Read the model definition and answer for the solid it produces. Units are mm, in the model's axes. Coordinates: 2 decimals unless noted, no trailing zeros. Order: outer loops, then holes, each group sorted by start corner. A loop starts at its lowest first (then second) coordinate and runs counter-clockwise, first axis right, second up.
from build123d import *

# Parameters (mm, degrees)
SKETCH1_W           = 30
SKETCH1_H           = 75.2
SKETCH1_R           = 5.25
BOSS_EXTRUDE1_DEPTH = 2.5
FILLET1_R           = 2


with BuildPart() as part:
    # Sketch1 → Boss-Extrude1 (new, symmetric)
    with BuildSketch(Plane.XY):
        Rectangle(SKETCH1_W, SKETCH1_H)
        with Locations((0, 23.1)):
            Circle(SKETCH1_R, mode=Mode.SUBTRACT)
    extrude(amount=BOSS_EXTRUDE1_DEPTH, both=True)

    # Fillet1
    fillet1_edges = [part.edges().sort_by_distance(p)[0] for p in [
        (-15, 37.6, 0),
        (15, 37.6, 0),
    ]]
    fillet(fillet1_edges, radius=FILLET1_R)


solid = part.part
Q1. This flat-tipped pin is pushed along its axis until it touches: P1, Ø6, axis at x = -1.5, y = 24, coming from the -Z side. Where does it stop, or does it pass through?
Q2. The part is cut by section C-C, the plane x = 0. Determine the outline of the cut face in (y, z).
Q3. Determine the mould class of faces 1 (the cylindrical face through (2.82, 27.53, -0.04)), 2 (the flat face through (0, 1, 2.5)), 3 (the cylindrical face through (14.43, 37, -0.04)) for opening direction X: +X half, -X half, draft (parallel to the pull), parting line (faces both ways), or undercut.
Q4. Straight lines are drawn through the part: L1, parallel to Y at x = 0, z = -0.25; L2, parallel to Y at x = -2.75, z = -1.6. For each, find the intervals that lie inside material, in ascending order.
Q5. The part is cut by section A-A, the plane z = -0.15. Determine the outline of the cut face in (x, y), then the cut area to 3 significant figures.
Q6. The part is cut by section B-B, the plane y = 23.1. Determine the outline of the cut face in (x, z), then the cut area to 3 significant figures.
Computed values:
1. P1: passes through
2. outline: (-37.6, -2.5) - (17.85, -2.5) - (17.85, 2.5) - (-37.6, 2.5) - close; (28.35, -2.5) - (37.6, -2.5) - (37.6, 2.5) - (28.35, 2.5) - close
3. face 1: undercut
3. face 2: draft
3. face 3: +X half
4. L1: y = -37.6 to 17.85, 28.35 to 37.6
4. L2: y = -37.6 to 18.63, 27.57 to 37.6
5. outline: (-15, -37.6) - (15, -37.6) - (15, 35.6) arc R2 ccw to (13, 37.6) - (-13, 37.6) arc R2 ccw to (-15, 35.6) - close; hole circle Ø10.5 at (0, 23.1)
5. area: 2,170 mm2
6. outline: (-15, -2.5) - (-5.25, -2.5) - (-5.25, 2.5) - (-15, 2.5) - close; (5.25, -2.5) - (15, -2.5) - (15, 2.5) - (5.25, 2.5) - close
6. area: 97.5 mm2
